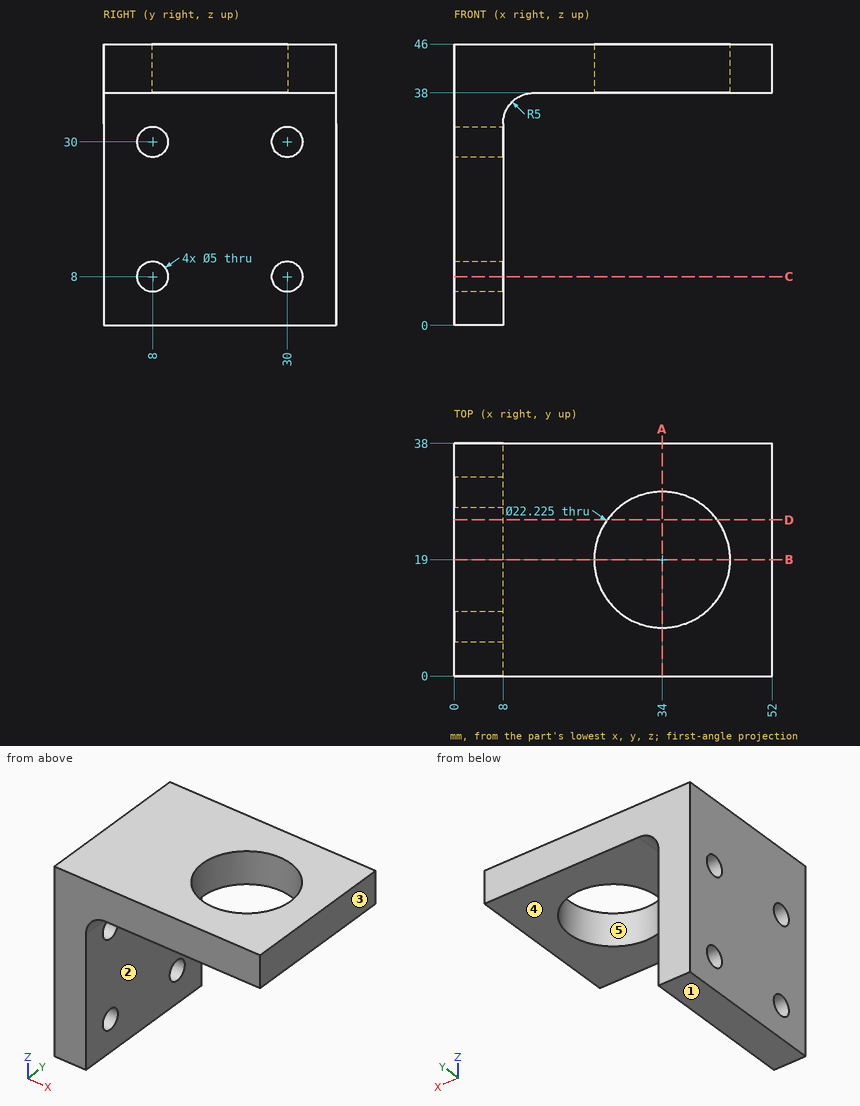
Verification items for this drawing (mm, ordinates from the low corner). A direction names the side the tool comes from. Round coordinates to 2 decimals unless told otherwise and drop trailing zeros. Loops run counter-clockwise (first coordinate to the right, second up) from the corner with the lowest first, then second, coordinate; pieces in that order, holes last. Notation, with made-up numbers: M 49.5,-2.75 L 80.5,-2.75 A8 ccw 80.5,4.25 Z; hole C -1,3.5 d4. An arc over 180 degrees is marked long. Answer as a JSON object with one key per item and string values.
1. Section check C-C (z = 8). Record the boundary of the cut face in (x, y).
Reply:
{"outline": "M 0,0 L 8,0 L 8,5.5 L 0,5.5 Z; M 0,10.5 L 8,10.5 L 8,27.5 L 0,27.5 Z; M 0,32.5 L 8,32.5 L 8,38 L 0,38 Z"}
2. Scan lines: line 1 (Y direction, x = 3.5, z = 8); line 2 (Y direction, x = 34, z = 44); line 3 (X direction, y = 27.5, z = 11.5). Record each from-to range of solid material in increasing order.
Reply:
{"line 1": "y = 0 to 5.5, 10.5 to 27.5, 32.5 to 38", "line 2": "y = 0 to 7.89, 30.11 to 38", "line 3": "x = 0 to 8"}
3. Gauge pin test, flat ends, axial feed: P1, Ø3, axis at y = 30, z = 8, coming from the +X side; P2, Ø8, axis at x = 25, y = 10, coming from the -Z side; P3, Ø3, axis at y = 16.5, z = 11, coming from the +X side. Record the tip position at first contact, or that the pin passes through.
Reply:
{"P1": "passes through", "P2": "stops at z = 38", "P3": "stops at x = 8"}
4. Mould release check, pull along X, two halves, no side actions. Record for the marked faces 3, 4 and 5: pulls with the +X half, pulls with the -X half, needs draft (parallel to the pull), parting line crosses it, or undercut.
Reply:
{"face 3": "pulls with the +X half", "face 4": "needs draft", "face 5": "undercut"}
5. Section check A-A (x = 34). Record the boundary of the cut face in (y, z).
Reply:
{"outline": "M 0,38 L 7.89,38 L 7.89,46 L 0,46 Z; M 30.11,38 L 38,38 L 38,46 L 30.11,46 Z"}
6. Section check D-D (y = 25.5). Record the boundary of the cut face in (x, z), plus the area to 3 significant figures.
Reply:
{"outline": "M 0,0 L 8,0 L 8,33 A5 cw 13,38 L 24.99,38 L 24.99,46 L 0,46 Z; M 43.01,38 L 52,38 L 52,46 L 43.01,46 Z", "area": "581 mm²"}
7. Access from +Z, -Z, +X, -X, +Y, -Y to the whole of each face (thin tool, end or side, straight path). Record for the marked faces 1 and 2.
Reply:
{"face 1": "-Z, +X, -X, +Y, -Y", "face 2": "-Z, +X, +Y, -Y"}
8. Section check B-B (y = 19). Record the boundary of the cut face in (x, z), plus the area to 3 significant figures.
Reply:
{"outline": "M 0,0 L 8,0 L 8,33 A5 cw 13,38 L 22.89,38 L 22.89,46 L 0,46 Z; M 45.11,38 L 52,38 L 52,46 L 45.11,46 Z", "area": "548 mm²"}
